The model under review builds one solid part; all positions refer to its coordinate system, in mm. A direction names the side the tool comes from. Round coordinates to 2 decimals unless told otherwise and drop trailing zeros. Write each loop counter-clockwise with the first axis right and the second up, starting at its lowest first coordinate (ties: lowest second). Pieces come first, ordered by that corner, then holes. Notation, with made-up numbers: M -16.5,-26.5 L -3.5,-26.5 A15 ccw -3.5,-1.5 Z; hole C 13.5,68.5 d10. An arc over 180 degrees is marked long. One line per item, written item: value. Start each with the question number.
1) For P1, Ø2, axis at x = 0, y = 0, coming from the -Z side; P2, Ø5, axis at y = -11.5, z = 6.5, coming from the +X side; P3, Ø4, axis at x = -22.5, z = 8, coming from the -Y side; P4, Ø4, axis at y = -15, z = 10, coming from the -X side, all flat-tipped, find the tip position at first contact; note any pin that passes through.
2) Take a section at B-B, the plane y = 6.5. Write out the cut boundary in (x, z), and give its area (3 significant figures).
3) Tool access review of faces 5 (the face through (13.336, -6.662, 5.916)), 6 (the face through (0, -2, 12)): name each direction out of +Z, -Z, +X, -X, +Y, -Y from which nothing blocks a thin tool from reaching the whole face with its end or side.
4) Wall thickness on probe 1 along Y at (x, z) = (19.5, 7.25); probe 2 along X at (y, z) = (-15, 0.75); probe 3 along X at (y, z) = (16.5, 4.25): over which ranges is each line inside the solid? List them lowest first.
5) Take a section at A-A, the plane x = 6.5. Write out the cut boundary in (y, z), and give its area (3 significant figures).
6) Take a section at D-D, the plane x = -21. Write out the cut boundary in (y, z).
7) Mouldability with a two-part tool opening along Y and no side actions: class faces 1 (the face through (-27.147, 6.86, 5.916)), 2 (the face through (0, -2, 0)), 3 (the face through (-6.787, 13.674, 5.916)), 4 (the face through (-29.97, 1.32, 5.92)) as +Y half, -Y half, draft (parallel to the pull), parting line (faces both ways), or undercut.
8) Take a section at C-C, the plane z = 9. Write out the cut boundary in (x, y), and give its area (3 significant figures).
from build123d import *

# Parameters (mm, degrees)
SKETCH2_R           = 30
BOSS_EXTRUDE1_DEPTH = 12
SKETCH4_R           = 1.25
CUT_EXTRUDE1_DEPTH  = 45.09081537


with BuildPart() as part:
    # Sketch2 → Boss-Extrude1 (new body)
    with BuildSketch(Plane.XY):
        Circle(SKETCH2_R)
        with BuildLine():
            Line((-10.13235825, 26.102400585), (-3.347071467, 0.892811622))
            Line((-3.347071467, 0.892811622), (-21.786572537, -17.588213585))
            ThreePointArc((-21.786572537, -17.588213585), (-27.054056577, 7.216510426), (-10.13235825, 26.102400585))
        make_face(mode=Mode.SUBTRACT)
        with BuildLine():
            Line((-17.539162882, -21.826079937), (0.900338188, -3.34505473))
            Line((0.900338188, -3.34505473), (26.12512604, -10.073618486))
            ThreePointArc((26.12512604, -10.073618486), (7.277346933, -27.037755484), (-17.539162882, -21.826079937))
        make_face(mode=Mode.SUBTRACT)
        with BuildLine():
            Line((-4.338553503, 27.661832071), (2.446733279, 2.452243108))
            Line((2.446733279, 2.452243108), (27.671521131, -4.276320648))
            ThreePointArc((27.671521131, -4.276320648), (19.776709644, 19.821245058), (-4.338553503, 27.661832071))
        make_face(mode=Mode.SUBTRACT)
    extrude(amount=BOSS_EXTRUDE1_DEPTH)

    # Sketch4 → Cut-Extrude1 (cut, through all)
    with BuildSketch(Plane.XY.offset(12)):
        Circle(SKETCH4_R)
    extrude(amount=-CUT_EXTRUDE1_DEPTH, mode=Mode.SUBTRACT)


solid = part.part
Checked values:
1. P1: passes through
1. P2: stops at x = 28.62
1. P3: stops at y = -21.9
1. P4: stops at x = -27.04
2. outline: M -29.29,0 L -27.24,0 L -27.24,12 L -29.29,12 Z; M -4.86,0 L 1.36,0 L 1.36,12 L -4.86,12 Z; M 27.24,0 L 29.29,0 L 29.29,12 L 27.24,12 Z
2. area: 124 mm2
3. face 5: +Z, -Z
3. face 6: +Z, +X, -X, +Y, -Y
4. probe 1: y = -22.8 to -20.09, -8.31 to -2.1, 20.09 to 22.8
4. probe 2: x = -25.98 to -23.64, -19.2 to -10.73, 23.64 to 25.98
4. probe 3: x = -25.05 to -22.62, -7.55 to -1.33, 22.62 to 25.05
5. outline: M -29.29,0 L -27.24,0 L -27.24,12 L -29.29,12 Z; M -4.84,0 L 1.37,0 L 1.37,12 L -4.84,12 Z; M 27.24,0 L 29.29,0 L 29.29,12 L 27.24,12 Z
5. area: 124 mm2
6. outline: M -21.42,0 L -16.8,0 L -16.8,12 L -21.42,12 Z; M 18.52,0 L 21.42,0 L 21.42,12 L 18.52,12 Z
7. face 1: undercut
7. face 2: draft
7. face 3: undercut
7. face 4: parting line
8. outline: C 0,0 d60; hole M -21.79,-17.59 L -3.35,0.89 L -10.13,26.1 A28 ccw Z; hole M -17.54,-21.83 A28 ccw 26.13,-10.07 L 0.9,-3.35 Z; hole M -4.34,27.66 L 2.45,2.45 L 27.67,-4.28 A28 ccw Z; hole C 0,0 d2.5
8. area: 847 mm2
